Read the model definition and answer for the solid it produces. Units are mm, in the model's axes. Round coordinates to 2 decimals unless told otherwise and drop trailing zeros. Return JSON: item names as keys, results as strings. Group by question number.
(1) A cutting plane is placed at A-A on y = -221. State how many separate pieces and enclosed holes the cut face has, then the cut area to 3 significant figures.
(2) Given pin 1 (1 mm diameter, centred on x = -6.5, z = -6, fed in from +Y); pin 2 (1.9 mm diameter, centred on x = 3, y = -174, fed in from +Z); pin 3 (1.5 mm diameter, centred on x = -0.5, y = -293.5, fed in from -Z); pin 4 (3 mm diameter, centred on y = -257.5, z = -2.5, fed in from -X), each flat-ended and moving along its own axis, determine where each tip first touches the part or whether it passes through.
(3) Straight lines are drawn through the part: line 1 (Z direction, x = -10, y = -150); line 2 (X direction, y = -242.5, z = -11); line 3 (Z direction, x = 13.5, y = -369). For each, find the intervals that lie inside material, in ascending order.
```python
from build123d import *

# Parameters (mm, degrees)
F2_DEPTH = 400
F1_R     = 3.7
F1_W     = 4
F1_H     = 4
F3_DEPTH = 400.001


with BuildPart() as f2:
    # F0 (on Front) → F2 (new body)
    with BuildSketch(Plane.XZ):
        Polygon((-4.091443, 14.818899), (-14.491443, 14.818899), (-14.491443, 4.418899), (-13.991443, 4.418899), (-13.991443, 3.918899), (-12.291443, 3.918899), (-12.291443, 8.218899), (-9.291443, 8.218899), (-5.241443, 4.168899), (-5.241443, 0.318899), (-4.741443, -0.181101), (-5.241443, -0.681101), (-5.241443, -4.531101), (-9.291443, -8.581101), (-12.291443, -8.581101), (-12.291443, -4.281101), (-13.991443, -4.281101), (-13.991443, -4.781101), (-14.491443, -4.781101), (-14.491443, -15.181101), (-4.091443, -15.181101), (-4.091443, -14.681101), (-3.591443, -14.681101), (-3.591443, -12.981101), (-7.891443, -12.981101), (-7.891443, -9.981101), (-3.841443, -5.931101), (0.008557, -5.931101), (0.508557, -5.431101), (1.008557, -5.931101), (4.858557, -5.931101), (8.908557, -9.981101), (8.908557, -12.981101), (4.608557, -12.981101), (4.608557, -14.681101), (5.108532, -14.681101), (5.108532, -15.181101), (15.508557, -15.181101), (15.508557, -4.781101), (15.008557, -4.781101), (15.008557, -4.281101), (13.308557, -4.281101), (13.308557, -8.581101), (10.308557, -8.581101), (6.258557, -4.531101), (6.258557, -0.681101), (5.758557, -0.181101), (6.258557, 0.318899), (6.258557, 4.168899), (10.308557, 8.218899), (13.308557, 8.218899), (13.308557, 3.918899), (15.008557, 3.918899), (15.008557, 4.418899), (15.508557, 4.418899), (15.508557, 14.818899), (5.108532, 14.818899), (5.108532, 14.318899), (4.608557, 14.323857), (4.608557, 12.623857), (8.908557, 12.623857), (8.908557, 9.623857), (4.853598, 5.568899), (1.003598, 5.568899), (0.508557, 5.068899), (0.003549, 5.568899), (-3.846451, 5.568899), (-7.891443, 9.618899), (-7.891443, 12.618899), (-3.591443, 12.618899), (-3.591443, 14.318899), (-4.091443, 14.318899), align=None)
    extrude(amount=F2_DEPTH)

    # F1 (on Front) → F3 (cut, through all)
    with BuildSketch(Plane.XZ):
        with Locations((0.508557, -0.181101)):
            Circle(F1_R)
        with Locations((12.228557, 11.538899)):
            Rectangle(F1_W, F1_H)
        with Locations((12.228557, -11.901101)):
            Rectangle(F1_W, F1_H)
        with Locations((-11.211443, -11.901101)):
            Rectangle(F1_W, F1_H)
        with Locations((-11.211443, 11.53863)):
            Rectangle(F1_W, F1_H)
    extrude(amount=F3_DEPTH, mode=Mode.SUBTRACT)


solid = f2.part
```
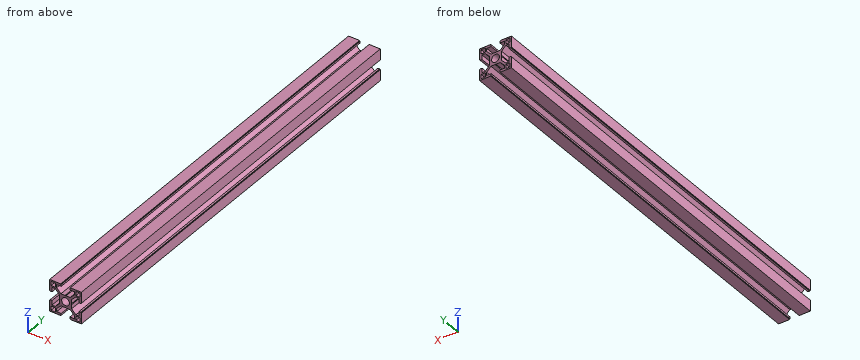
Checks:
{
 "1": {"separate pieces": "1", "enclosed holes": "5", "area": "310 mm^2"},
 "2": {"pin 1": "stops at y = 0", "pin 2": "stops at z = 5.57", "pin 3": "stops at z = -5.93", "pin 4": "stops at x = -5.24"},
 "3": {"line 1": "z = -15.18 to -13.9, -9.9 to -8.58, 8.22 to 9.54, 13.54 to 14.82", "line 2": "x = -14.49 to -13.21, -9.21 to -7.89, 8.91 to 10.23, 14.23 to 15.51", "line 3": "z = -15.18 to -13.9, -9.9 to -4.28, 3.92 to 9.54, 13.54 to 14.82"}
}
